```python
from build123d import *

# Parameters (mm, degrees)
BOSS_EXTRUDE1_DEPTH = 4.5
CUT_EXTRUDE1_START  = -3
CUT_EXTRUDE1_DEPTH  = 1.5
BOSS_EXTRUDE2_DEPTH = 1.5


with BuildPart() as part:
    # Sketch1 → Boss-Extrude1 (new body)
    with BuildSketch(Plane(origin=(0, 0, 0), x_dir=(1, 0, 0), z_dir=(0, 1, 0))):
        with BuildLine():
            Line((0, 0), (5, 0))
            ThreePointArc((5, 0), (3.535533906, -3.535533906), (0, -5))
            Line((0, -5), (0, 0))
        make_face()
    extrude(amount=BOSS_EXTRUDE1_DEPTH)

    # Sketch2 → Cut-Extrude1 (cut)
    with BuildSketch(Plane(origin=(0, 4.5, 0), x_dir=(1, 0, 0), z_dir=(0, 1, 0)).offset(CUT_EXTRUDE1_START)):
        with BuildLine():
            Line((4.822051432, -1.322051432), (1.322051432, -1.322051432))
            Line((1.322051432, -1.322051432), (1.322051432, -4.822051432))
            ThreePointArc((1.322051432, -4.822051432), (3.535533906, -3.535533906), (4.822051432, -1.322051432))
        make_face()
    extrude(amount=CUT_EXTRUDE1_DEPTH, mode=Mode.SUBTRACT)

    # Sketch3 → Boss-Extrude2 (add)
    with BuildSketch(Plane(origin=(0, 4.5, 0), x_dir=(1, 0, 0), z_dir=(0, 1, 0))):
        with BuildLine():
            Line((4.898979486, -1), (1, -1))
            Line((1, -1), (1, -4.898979486))
            ThreePointArc((1, -4.898979486), (0.50254481, -4.974680765), (0, -5))
            Line((0, -5), (0, 0))
            Line((0, 0), (5, 0))
            ThreePointArc((5, 0), (4.974680765, -0.50254481), (4.898979486, -1))
        make_face()
    extrude(amount=BOSS_EXTRUDE2_DEPTH)


solid = part.part
```
Model file for the job. Use its own axes, mm. A direction names the side the tool comes from. Round coordinates to 2 decimals unless told otherwise and drop trailing zeros. Write each loop counter-clockwise with the first axis right and the second up, starting at its lowest first coordinate (ties: lowest second). Pieces come first, ordered by that corner, then holes. Notation, with made-up numbers: M 10,32.25 L 28,32.25 A23 ccw 28,47.25 Z; hole C 26.5,39.5 d7. An arc over 180 degrees is marked long. Put each result on its own line as item: value.
Item 1: Cut at C-C (z = 2.4). List the corners of the cut face in (x, y), and give its area (3 significant figures).
Responses:
outline: M 0,0 L 4.39,0 L 4.39,1.5 L 1.32,1.5 L 1.32,3 L 4.39,3 L 4.39,4.5 L 1,4.5 L 1,6 L 0,6 Z
area: 16.6 mm²
Item 2: Cut at B-B (x = 3.9). List the corners of the cut face in (y, z).
Responses:
outline: M 0,0 L 6,0 L 6,1 L 4.5,1 L 4.5,3.13 L 3,3.13 L 3,1.32 L 1.5,1.32 L 1.5,3.13 L 0,3.13 Z
Item 3: Flat gauge pins, fed straight in: P1, Ø2, axis at y = 2, z = 1, coming from the +X side; P2, Ø2, axis at x = 3, y = 0.5, coming from the +Z side; P3, Ø1.6, axis at x = 3, y = 5, coming from the +Z side; P4, Ø1.2, axis at x = 3.5, z = 2.5, coming from the +Y side. Where does each tip first touch, or does it go through?
Responses:
P1: x = 5
P2: z = 4.58
P3: z = 4.4
P4: y = 4.5
Item 4: Cut at A-A (y = 2.4). List the corners of the cut face in (x, z).
Responses:
outline: M 0,0 L 5,0 A5 ccw 4.82,1.32 L 1.32,1.32 L 1.32,4.82 A5 ccw 0,5 Z
Item 5: Mould opens along Y. For faces 4 (the flat face through (0, 3, 3)), 5 (the flat face through (3, 1.5, 3)), 6 (the flat face through (3, 3, 3)), 7 (the flat face through (2, 0, 2)) say: +Y half, -Y half, draft (parallel to the pull), parting line (faces both ways), or undercut.
Responses:
face 4: draft
face 5: undercut
face 6: undercut
face 7: -Y half
Item 6: Cut at D-D (y = 4.65). List the corners of the cut face in (x, z), and give its area (3 significant figures).
Responses:
outline: M 0,0 L 5,0 A5 ccw 4.9,1 L 1,1 L 1,4.9 A5 ccw 0,5 Z
area: 8.93 mm²
Item 7: Tool access for faces 1 (the flat face through (2, 3, 0)), 2 (the flat face through (3, 2, 1.322)), 3 (the flat face through (1, 5, 3)): list every direction of +Z, -Z, +X, -X, +Y, -Y with a clear straight run to the whole face (end or side of a thin tool).
Responses:
face 1: -Z, +X, -X, +Y, -Y
face 2: +Z, +X
face 3: +Z, +X, +Y
Item 8: Probe L1, parallel to Y at x = 2.3, z = 3.4; L2, parallel to Z at x = 4, y = 5.75; L3, parallel to Z at x = 1, y = 2.6. List the from-to ranges inside material, lowest first. Write a range as from..to.
Responses:
L1: 0..1.5, 3..4.5
L2: 0..1
L3: 0..4.9
